Input: part model. Units: mm. Frame: model coordinates. A direction names the side the tool comes from. Coordinates: 2 decimals unless noted, no trailing zeros. Loops run counter-clockwise (first coordinate to the right, second up) from the corner with the lowest first, then second, coordinate; pieces in that order, holes last.
(1) Section C-C, the plane y = 0. Return loops of the section in (x, z), then the cut area to 3 significant figures.
(2) Contact query for flat-ended pins moving along their axis: P1, Ø1.1, axis at x = 2, z = 3, coming from the +Y side; P2, Ø2.5, axis at x = -6, z = 2.5, coming from the +Y side; P3, Ø0.7, axis at y = 36, z = 3, coming from the -X side. Output: stop coordinate, or through.
(3) Section A-A, the plane y = 26. Return loops of the section in (x, z) (3 decimals), then the cut area to 3 significant figures.
(4) Mould query, pull axis X, two halves, no side actions, for faces 4 (the face through (0.6, 36, 3)), 5 (the face through (-2.36, 13.75, 3.2)), 6 (the face through (-9.715, -9.699, 2.532)), 7 (the face through (9.61, -9.62, 4.88)). Classes: released by +X, released by -X, zero draft, split by the parting line, or undercut.
(5) Section B-B, the plane z = 3.95. Return loops of the section in (x, y) (3 decimals).
(6) Line query: L1, parallel to X at y = 27, z = 0.3; L2, parallel to Y at x = -2, z = 4.4; L3, parallel to X at y = 0, z = 0.9. Output: solid intervals per line, ascending.
(7) Set-up query: faces 1 (the face through (-1.75, 26, 1)), 2 (the face through (-7.925, 27, 3)), 3 (the face through (-9.62, -9.61, 4.88)). Return all of +Z, -Z, +X, -X, +Y, -Y with unobstructed straight access to the full face (end or side cutting, diameter ignored); none if empty.
```python
from build123d import *

# Parameters (mm, degrees)
SKETCH1_R           = 2.75
BOSS_EXTRUDE1_DEPTH = 5
CUT_EXTRUDE1_REACH  = 46.43
SKETCH5_R           = 1.45
SKETCH6_R           = 1.45
CUT_EXTRUDE2_DEPTH  = 3.4
SKETCH7_W           = 2.725
SKETCH7_H           = 16.25
CUT_EXTRUDE3_DEPTH  = 1.2
CUT_EXTRUDE4_REACH  = 46.278
SKETCH8_W           = 3.5
SKETCH8_H           = 5.5
FILLET1_R           = 1
FILLET3_R           = 0.25
CHAMFER2_SIZE       = 0.25


with BuildPart() as part:
    # Sketch1 → Boss-Extrude1 (new body)
    with BuildSketch(Plane.XY):
        with BuildLine():
            ThreePointArc((10, 33), (0, 43), (-10, 33))
            Line((-10, 33), (-10, -10))
            Line((-10, -10), (10, -10))
            Line((10, -10), (10, 33))
        make_face()
        Circle(SKETCH1_R, mode=Mode.SUBTRACT)
    extrude(amount=BOSS_EXTRUDE1_DEPTH)

    # Sketch4 → CSK for M5 Flat Head Machine Screw1 (revolve, cut)
    with BuildSketch(Plane(origin=(0, 0, 5), x_dir=(0, -1, 0), z_dir=(1, 0, 0))):
        Polygon((0, 0), (0, 5), (2.75, 5), (2.75, 2.75), (5, 0.5), (5, 0), align=None)
    revolve(axis=Axis((0, 0, 11.35), (0, 0, -1)), mode=Mode.SUBTRACT)

    # Sketch5 → Cut-Extrude1 (cut, up to next)
    with BuildSketch(Plane.XY.offset(5), mode=Mode.PRIVATE) as cut_extrude1_sk1:
        with Locations((-2.3, 36.35)):
            Circle(SKETCH5_R)
    cut_extrude1_tool1 = extrude(cut_extrude1_sk1.sketch, amount=-CUT_EXTRUDE1_REACH, mode=Mode.PRIVATE) & part.part
    # Sketch5 → Cut-Extrude1 (cut, up to next)
    with BuildSketch(Plane.XY.offset(5), mode=Mode.PRIVATE) as cut_extrude1_sk2:
        with Locations((-2.3, 16.65)):
            Circle(SKETCH5_R)
    cut_extrude1_tool2 = extrude(cut_extrude1_sk2.sketch, amount=-CUT_EXTRUDE1_REACH, mode=Mode.PRIVATE) & part.part
    add(cut_extrude1_tool1.solids().sort_by_distance((-2.3, 36.35, 5))[0], mode=Mode.SUBTRACT)
    add(cut_extrude1_tool2.solids().sort_by_distance((-2.3, 16.65, 5))[0], mode=Mode.SUBTRACT)

    # Sketch6 → Cut-Extrude2 (cut)
    with BuildSketch(Plane.XY.offset(5)):
        with BuildLine():
            Line((3.325, 34.625), (0.6, 34.625))
            Line((0.6, 34.625), (0.6, 36.35))
            ThreePointArc((0.6, 36.35), (-2.3, 39.25), (-5.2, 36.35))
            Line((-5.2, 36.35), (-5.2, 34.625))
            Line((-5.2, 34.625), (-7.925, 34.625))
            Line((-7.925, 34.625), (-7.925, 18.375))
            Line((-7.925, 18.375), (-5.2, 18.375))
            Line((-5.2, 18.375), (-5.2, 16.65))
            ThreePointArc((-5.2, 16.65), (-2.3, 13.75), (0.6, 16.65))
            Line((0.6, 16.65), (0.6, 18.375))
            Line((0.6, 18.375), (3.325, 18.375))
            Line((3.325, 18.375), (3.325, 34.625))
        make_face()
        with Locations((-2.3, 36.35)):
            Circle(SKETCH6_R, mode=Mode.SUBTRACT)
        with Locations((-2.3, 16.65)):
            Circle(SKETCH6_R, mode=Mode.SUBTRACT)
    extrude(amount=-CUT_EXTRUDE2_DEPTH, mode=Mode.SUBTRACT)

    # Sketch7 → Cut-Extrude3 (cut)
    with BuildSketch(Plane.XY.offset(1.6)):
        with Locations((-6.5625, 26.5)):
            Rectangle(SKETCH7_W, SKETCH7_H)
    extrude(amount=-CUT_EXTRUDE3_DEPTH, mode=Mode.SUBTRACT)

    # Sketch8 → Cut-Extrude4 (cut, up to next)
    with BuildSketch(Plane.XY.offset(1.6), mode=Mode.PRIVATE) as cut_extrude4_sk1:
        with Locations((0, 26.5)):
            Rectangle(SKETCH8_W, SKETCH8_H)
    cut_extrude4_tool1 = extrude(cut_extrude4_sk1.sketch, amount=-CUT_EXTRUDE4_REACH, mode=Mode.PRIVATE) & part.part
    add(cut_extrude4_tool1.solids().sort_by_distance((0, 26.5, 1.6))[0], mode=Mode.SUBTRACT)

    # Fillet1
    fillet1_edges = [part.edges().sort_by_distance(p)[0] for p in [
        (10, -10, 2.5),
        (-10, -10, 2.5),
    ]]
    fillet(fillet1_edges, radius=FILLET1_R)

    # Fillet3
    fillet3_edges = [part.edges().sort_by_distance(p)[0] for p in [
        (1.75, 29.25, 0.8),
        (1.75, 23.75, 0.8),
        (-1.75, 23.75, 0.8),
        (-1.75, 29.25, 0.8),
        (0.6, 34.625, 3.3),
        (3.325, 34.625, 3.3),
        (3.325, 18.375, 3.3),
        (0.6, 18.375, 3.3),
        (-5.2, 18.375, 3.3),
        (-7.925, 18.375, 2.7),
        (-7.925, 34.625, 2.7),
        (-5.2, 34.625, 3.3),
        (-7.925, 26.5, 0.4),
        (-6.5625, 34.625, 0.4),
        (-5.2, 26.5, 0.4),
        (-6.5625, 18.375, 0.4),
    ]]
    fillet(fillet3_edges, radius=FILLET3_R)

    # Chamfer2
    chamfer2_edges = [part.edges().sort_by_distance(p)[0] for p in [
        (0, 43, 5),
        (0, -10, 0),
        (-9.707106781, -9.707106781, 0),
        (9.707106781, -9.707106781, 0),
        (0, -10, 5),
        (-9.707106781, -9.707106781, 5),
        (9.707106781, -9.707106781, 5),
        (-6.5625, 34.625, 5),
        (-6.5625, 18.375, 5),
        (-7.925, 26.5, 5),
        (1.9625, 34.625, 5),
        (3.325, 26.5, 5),
        (1.9625, 18.375, 5),
        (1.75, 26.5, 1.6),
        (0, 23.75, 1.6),
        (-1.75, 26.5, 1.6),
        (0, 29.25, 1.6),
        (-1.75, 26.5, 0),
        (0, 29.25, 0),
        (-10, 12, 5),
        (1.75, 26.5, 0),
        (0, 23.75, 0),
        (-7.851776695, 34.551776695, 5),
        (-7.851776695, 18.448223305, 5),
        (3.251776695, 18.448223305, 5),
        (3.251776695, 34.551776695, 5),
        (-1.676776695, 29.176776695, 1.6),
        (-1.676776695, 29.176776695, 0),
        (1.676776695, 29.176776695, 1.6),
        (1.676776695, 29.176776695, 0),
        (1.676776695, 23.823223305, 1.6),
        (1.676776695, 23.823223305, 0),
        (-1.676776695, 23.823223305, 1.6),
        (-1.676776695, 23.823223305, 0),
        (-3.75, 36.35, 0),
        (-3.75, 16.65, 0),
        (-5.2, 17.3875, 5),
        (-3.75, 36.35, 1.6),
        (0.6, 35.6125, 5),
        (-3.75, 16.65, 1.6),
        (-2.3, 39.25, 5),
        (-5.2, 35.6125, 5),
        (-2.3, 13.75, 5),
        (0.6, 17.3875, 5),
        (10, 12, 5),
        (-2.75, 0, 0),
        (-10, 12, 0),
        (0, 43, 0),
        (10, 12, 0),
    ]]
    chamfer(chamfer2_edges, length=CHAMFER2_SIZE)


solid = part.part
```
Report:
1. outline: (-10, 0.25) - (-9.75, 0) - (-3, 0) - (-2.75, 0.25) - (-2.75, 2.25) - (-5, 4.5) - (-5, 5) - (-9.75, 5) - (-10, 4.75) - close; (2.75, 0.25) - (3, 0) - (9.75, 0) - (10, 0.25) - (10, 4.75) - (9.75, 5) - (5, 5) - (5, 4.5) - (2.75, 2.25) - close
1. area: 65.0 mm2
2. P1: stops at y = 42.89
2. P2: stops at y = 41.8
2. P3: stops at x = -9.64
3. outline: (-10, 0.25) - (-9.75, 0) - (-2, 0) - (-1.75, 0.25) - (-1.75, 1.35) - (-2, 1.6) - (-5.2, 1.6) - (-5.2, 0.65) arc R0.25 cw to (-5.45, 0.4) - (-7.675, 0.4) arc R0.25 cw to (-7.925, 0.65) - (-7.925, 4.75) - (-8.175, 5) - (-9.75, 5) - (-10, 4.75) - close; (1.75, 0.25) - (2, 0) - (9.75, 0) - (10, 0.25) - (10, 4.75) - (9.75, 5) - (3.575, 5) - (3.325, 4.75) - (3.325, 1.6) - (2, 1.6) - (1.75, 1.35) - close
3. area: 52.6 mm2
4. face 4: undercut
4. face 5: undercut
4. face 6: released by -X
4. face 7: released by +X
5. outline: (-10, -9) arc R1 ccw to (-9, -10) - (9, -10) arc R1 ccw to (10, -9) - (10, 33) arc R10 ccw to (-10, 33) - close; hole (-7.925, 18.625) arc R0.25 ccw to (-7.675, 18.375) - (-5.45, 18.375) arc R0.25 cw to (-5.2, 18.125) - (-5.2, 16.65) arc R2.9 ccw to (0.6, 16.65) - (0.6, 18.125) arc R0.25 cw to (0.85, 18.375) - (3.075, 18.375) arc R0.25 ccw to (3.325, 18.625) - (3.325, 34.375) arc R0.25 ccw to (3.075, 34.625) - (0.85, 34.625) arc R0.25 cw to (0.6, 34.875) - (0.6, 36.35) arc R2.9 ccw to (-5.2, 36.35) - (-5.2, 34.875) arc R0.25 cw to (-5.45, 34.625) - (-7.675, 34.625) arc R0.25 ccw to (-7.925, 34.375) - close; hole circle Ø8.9 at (0, 0)
6. L1: x = -10 to -1.75, 1.75 to 10
6. L2: y = -10 to -4.47, 4.47 to 13.77, 39.23 to 42.8
6. L3: x = -10 to -2.75, 2.75 to 10
7. face 1: +Z, -Z
7. face 2: +Z
7. face 3: +Z, -X, -Y
